Design review of the part shown in the three views and the two pictorial views. Dimensions are in mm from the part's minimum x, y and z. A direction names the side the tool comes from. Give positions to 0.01 mm unless a question says otherwise; leave off trailing zeros. Write each loop counter-clockwise with the first axis right and the second up, starting at its lowest first coordinate (ties: lowest second). Pieces come first, ordered by that corner, then holes. Notation, with made-up numbers: (-4.5, 87.5) -> (37.5, 87.5) arc R24 ccw to (37.5, 99.5) -> close; hole circle Ø11 at (56.25, -17). An arc over 180 degrees is marked (long way). Use CSV: the item, a comma, the result in double quotes.
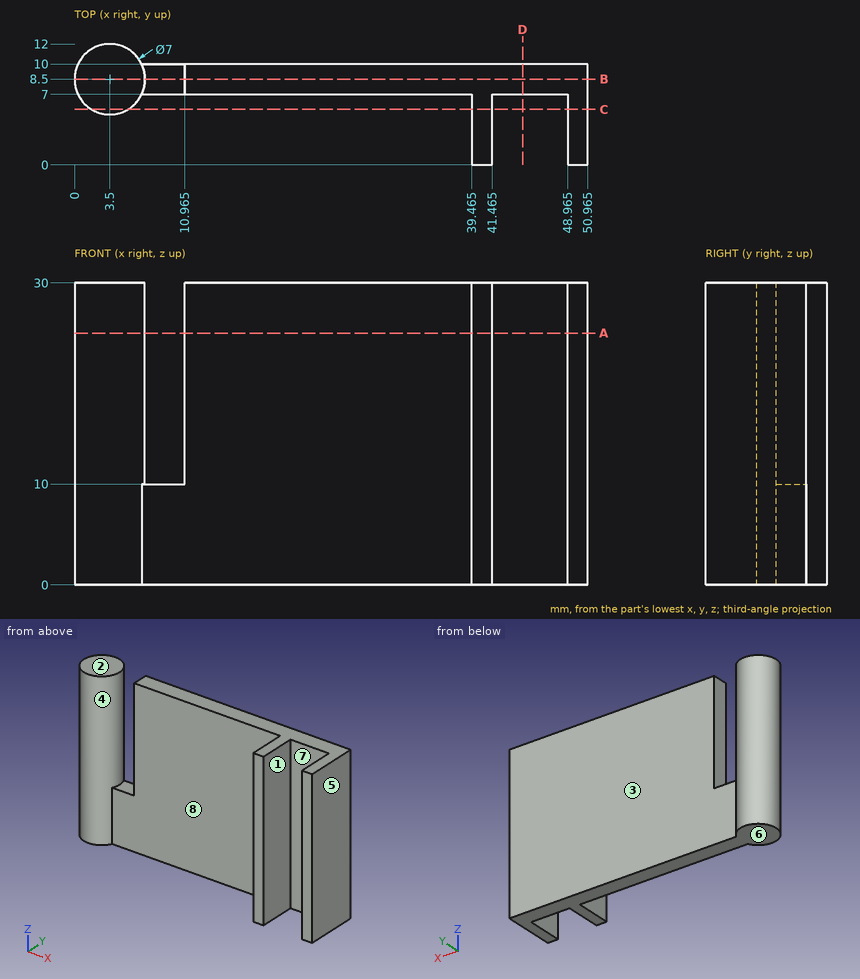
Q1. Machinability: for the marked faces 1, 2, 3 and 4, which of the approach directions +Z, -Z, +X, -X, +Y, -Y give a long, thin tool a straight path to every point of the face, cutting with its end or side? Answer none if there is none.
Derived:
face 1,"+Z, -Z, -Y"
face 2,"+Z, +X, -X, +Y, -Y"
face 3,"+Z, -Z, +X, +Y"
face 4,"+Z"
Q2. Insertion check: pin 1 (4 mm diameter, centred on x = 44, z = 9.5, fed in from -Y); pin 2 (9 mm diameter, centred on x = 35, z = 13, fed in from +Y); pin 3 (1 mm diameter, centred on y = 3, z = 23, fed in from -X) (3 decimals); pin 4 (4 mm diameter, centred on x = 37.5, y = 10.5, fed in from -Z). Each pin has a flat end and moves straight along its axis. Give the tip position at first contact, or say it passes through.
Derived:
pin 1,"stops at y = 7"
pin 2,"stops at y = 10"
pin 3,"stops at x = 39.465"
pin 4,"stops at z = 0"
Q3. Consider section D-D (x = 44.5). Write out the cut boundary in (y, z), then the cut area to 3 significant figures.
Derived:
outline,"(7, 0) -> (10, 0) -> (10, 30) -> (7, 30) -> close"
area,"90.0 mm2"
Q4. The part is to be moulded in two halves that separate along X. For the marked faces 5, 6, 7 and 8, say which applies: pulls with the +X half, pulls with the -X half, needs draft (parallel to the pull), parting line crosses it, or undercut.
Derived:
face 5,"pulls with the +X half"
face 6,"needs draft"
face 7,"undercut"
face 8,"undercut"
Q5. To check wall thickness, follow probe 1 along X at (y, z) = (3, 7) (3 decimals); probe 2 along Y at (x, z) = (23, 21.75); probe 3 along Y at (x, z) = (49, 8). State the ranges of each line that lie inside material, in increasing order.
Derived:
probe 1,"x = 39.465 to 41.465, 48.965 to 50.965"
probe 2,"y = 7 to 10"
probe 3,"y = 0 to 10"
Q6. Consider section C-C (y = 5.5). Write out the cut boundary in (x, z) (1 decimal).
Derived:
outline,"(1.7, 0) -> (5.3, 0) -> (5.3, 30) -> (1.7, 30) -> close; (39.5, 0) -> (41.5, 0) -> (41.5, 30) -> (39.5, 30) -> close; (49, 0) -> (51, 0) -> (51, 30) -> (49, 30) -> close"
Q7. Consider section B-B (y = 8.5). Write out the cut boundary in (x, z) (3 decimals).
Derived:
outline,"(0, 0) -> (50.965, 0) -> (50.965, 30) -> (10.965, 30) -> (10.965, 10) -> (7, 10) -> (7, 30) -> (0, 30) -> close"
Q8. Consider section A-A (z = 25). Write out the cut boundary in (x, y) (3 decimals).
Derived:
outline,"circle Ø7 at (3.5, 8.5); (10.965, 7) -> (39.465, 7) -> (39.465, 0) -> (41.465, 0) -> (41.465, 7) -> (48.965, 7) -> (48.965, 0) -> (50.965, 0) -> (50.965, 10) -> (10.965, 10) -> close"
